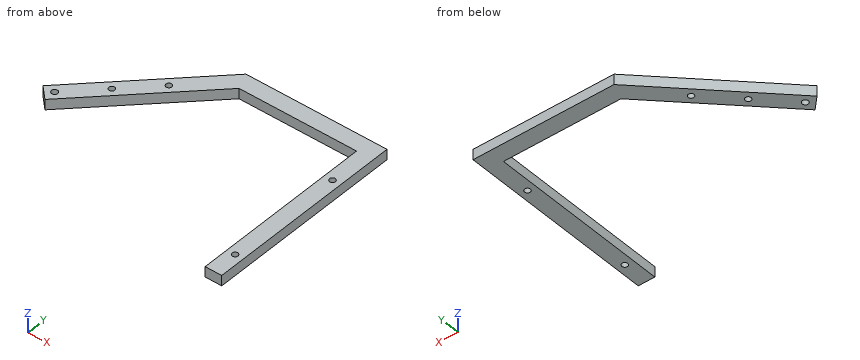
Autodesk Inventor part; units mm, degrees
ref_plane "YZ Plane" through (0, 0, 0) normal (1, 0, 0) x (0, 1, 0)
ref_plane "XZ Plane" through (0, 0, 0) normal (0, 1, 0) x (-1, 0, 0)
ref_plane "XY Plane" through (0, 0, 0) normal (0, 0, 1) x (1, 0, 0)
ref_plane "Arbeitsebene1" through (0, 0, 0) normal (0, 0, 1) x (1, 0, 0)
sketch "Skizze1" plane through (0, 0, 0) normal (0, 0, 1) x (1, 0, 0)
  circle A0 centre (41.3693, 78.2732) radius 1.4
  circle A1 centre (11.3693, 48.2732) radius 1.49
  line L0 (5.7124, 48.2732) -> (41.3693, 83.9301)
  line L1 (47.0261, 78.2732) -> (11.3693, 42.6164)
  line L2 (41.3693, 83.9301) -> (47.0261, 78.2732)
  line L3 (11.3693, 42.6164) -> (5.7124, 48.2732)
  line L4 (47.0261, 78.2732) -> (41.3693, 83.9301)
  line L5 (41.3693, 83.9301) -> (59.0469, 101.6077)
  line L6 (59.0469, 101.6077) -> (64.7038, 95.9509)
  line L7 (64.7038, 95.9509) -> (47.0261, 78.2732)
  line L8 (59.0469, 101.6077) -> (59.0469, 93.6077)
  line L9 (59.0469, 93.6077) -> (119.0469, 93.6077)
  line L10 (119.0469, 93.6077) -> (119.0469, 101.6077)
  line L11 (119.0469, 101.6077) -> (59.0469, 101.6077)
  line L12 (119.0469, 101.6077) -> (119.0469, 6.2524)
  line L13 (119.0469, 6.2524) -> (127.0469, 6.2524)
  line L14 (127.0469, 6.2524) -> (127.0469, 101.6077)
  line L15 (127.0469, 101.6077) -> (119.0469, 101.6077)
  circle A2 centre (26.3693, 63.2732) radius 1.4
  point P0 (0, 0)
  point P1 (62.3606, 93.6077)
  dimension "d0" = 25
  dimension "d1" = 8
  dimension "d2" = 60
  dimension "d3" = 8
  dimension "d10" = 2.8
extrude "Extrusion1" add sketch "Skizze1" along normal blind 5
sketch "Skizze2" plane through (0, 0, 5) normal (0, 0, 1) x (1, 0, 0)
  line L0 (127.0469, 6.2524) -> (127.0469, 101.6077)
  line L1 (127.0469, 101.6077) -> (59.0469, 101.6077)
  line L2 (59.0469, 101.6077) -> (5.7124, 48.2732)
  line L3 (5.7124, 48.2732) -> (11.3693, 42.6164)
  line L4 (11.3693, 42.6164) -> (62.3606, 93.6077)
  line L5 (62.3606, 93.6077) -> (119.0469, 93.6077)
  line L6 (119.0469, 93.6077) -> (119.0469, 6.2524)
  line L7 (119.0469, 6.2524) -> (127.0469, 6.2524)
  circle A0 centre (11.3693, 48.2732) radius 1.49
  circle A1 centre (41.3693, 78.2732) radius 1.4
  circle A2 centre (123.0469, 18.77) radius 1.4
  circle A3 centre (123.0469, 74.9405) radius 1.4
  point P0 (0, 0)
  dimension "d6" = 2.8
  dimension "d7" = 2.8
extrude "Extrusion2" cut sketch "Skizze2" against normal blind 5 contours A2 | A3
properties part number "NematostellaImager_illuminationmount"
Check sheet for the modelled part. Datum: model origin and axes. Units: mm. Give positions to 0.01 mm unless a question says otherwise; leave off trailing zeros. Loops run counter-clockwise (first coordinate to the right, second up) from the corner with the lowest first, then second, coordinate; pieces in that order, holes last. Notation, with made-up numbers: M 4,32.5 L 60,32.5 A14 ccw 60,55.5 Z; hole C 55,-4 d8. An arc over 180 degrees is marked long. Answer as CSV lines item,"result".
Item 1: Sectioned sample at D-D, the plane x = 71. Enter the section's corners in (y, z).
Reply:
outline,"M 93.61,0 L 101.61,0 L 101.61,5 L 93.61,5 Z"
Item 2: Sectioned sample at B-B, the plane z = 4.1. Enter the section's corners in (x, y).
Reply:
outline,"M 5.71,48.27 L 11.37,42.62 L 62.36,93.61 L 119.05,93.61 L 119.05,6.25 L 127.05,6.25 L 127.05,101.61 L 59.05,101.61 Z; hole C 11.37,48.27 d2.98; hole C 26.37,63.27 d2.8; hole C 41.37,78.27 d2.8; hole C 123.05,18.77 d2.8; hole C 123.05,74.94 d2.8"
Item 3: Scan lines: L1, parallel to X at y = 47.5, z = 2.7; L2, parallel to X at y = 73, z = 2.25; L3, parallel to X at y = 15, z = 3. Record each from-to range of solid material in increasing order.
Reply:
L1,"6.49 to 10.1, 12.64 to 16.25, 119.05 to 127.05"
L2,"30.44 to 41.75, 119.05 to 127.05"
L3,"119.05 to 127.05"
Item 4: Sectioned sample at C-C, the plane y = 53.5. Enter the section's corners in (x, z), then the cut area to 3 significant figures.
Reply:
outline,"M 10.94,0 L 22.25,0 L 22.25,5 L 10.94,5 Z; M 119.05,0 L 127.05,0 L 127.05,5 L 119.05,5 Z"
area,"96.6 mm^2"
Item 5: Depth check by flat-ended pin: pin 1 Ø1.7 at (x, y) = (123.05, 74.94) entering from -Z; pin 2 Ø1.5 at (x, z) = (78.5, 4) entering from -Y. Enter the tip coordinate at first touch or a pass-through.
Reply:
pin 1,"through"
pin 2,"y = 93.61"
Item 6: Sectioned sample at A-A, the plane y = 18.77. Enter the section's corners in (x, z).
Reply:
outline,"M 119.05,0 L 121.65,0 L 121.65,5 L 119.05,5 Z; M 124.45,0 L 127.05,0 L 127.05,5 L 124.45,5 Z"
